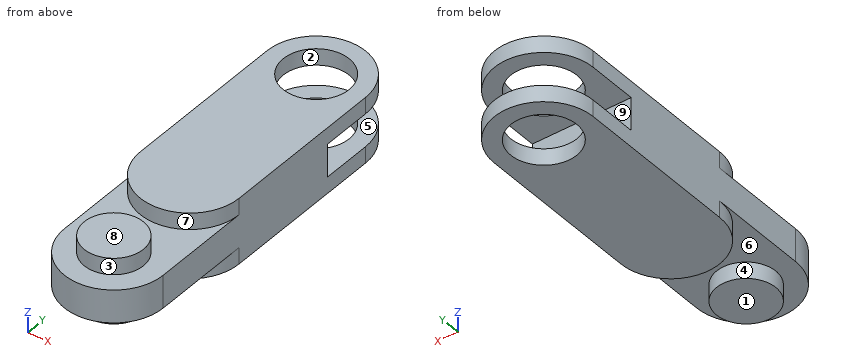
```python
from build123d import *

# Parameters (mm, degrees)
CROQUIS1_R                 = 10
SALIENTE_EXTRUIR1_DEPTH    = 10
CORTAR_EXTRUIR2_DEPTH      = 97.695398029
CORTAR_EXTRUIR2_DEPTH_BACK = 97.695398029
CROQUIS2_W                 = 10
CROQUIS2_H                 = 30
CORTAR_EXTRUIR4_START      = -5
CROQUIS4_R                 = 8.968507367
CORTAR_EXTRUIR4_DEPTH      = 92.695398029
CORTAR_EXTRUIR6_START      = 5
CROQUIS4_2_R               = 8.968507367
CORTAR_EXTRUIR6_DEPTH      = 92.695398029


with BuildPart() as part:
    # Croquis1 → Saliente-Extruir1 (new, symmetric)
    with BuildSketch(Plane.XY):
        with BuildLine():
            Line((-15, 0), (-15, 80))
            ThreePointArc((-15, 80), (0, 95), (15, 80))
            Line((15, 80), (15, 0))
            ThreePointArc((15, 0), (0, -15), (-15, 0))
        make_face()
        with Locations((0, 80)):
            Circle(CROQUIS1_R, mode=Mode.SUBTRACT)
    extrude(amount=SALIENTE_EXTRUIR1_DEPTH, both=True)

    # Croquis2 → Cortar-Extruir2 (cut, two sides: drawn at the far end of the back side and taken through both)
    with BuildSketch(Plane(origin=(0, 0, 0), x_dir=(0, 0, -1), z_dir=(1, 0, 0)).offset(-CORTAR_EXTRUIR2_DEPTH_BACK)):
        with Locations((0, 80)):
            Rectangle(CROQUIS2_W, CROQUIS2_H)
    extrude(amount=CORTAR_EXTRUIR2_DEPTH + CORTAR_EXTRUIR2_DEPTH_BACK, mode=Mode.SUBTRACT)

    # Croquis4 → Cortar-Extruir4 (cut, through all)
    with BuildSketch(Plane.XY.offset(CORTAR_EXTRUIR4_START)):
        with BuildLine():
            Line((-15, 30), (-15, 0))
            ThreePointArc((-15, 0), (0, -15), (15, 0))
            Line((15, 0), (15, 30))
            ThreePointArc((15, 30), (0, 15), (-15, 30))
        make_face()
        Circle(CROQUIS4_R, mode=Mode.SUBTRACT)
    extrude(amount=-CORTAR_EXTRUIR4_DEPTH, mode=Mode.SUBTRACT)

    # Croquis4<2> → Cortar-Extruir6 (cut, through all)
    with BuildSketch(Plane.XY.offset(CORTAR_EXTRUIR6_START)):
        with BuildLine():
            Line((-15, 30), (-15, 0))
            ThreePointArc((-15, 0), (0, -15), (15, 0))
            Line((15, 0), (15, 30))
            ThreePointArc((15, 30), (0, 15), (-15, 30))
        make_face()
        Circle(CROQUIS4_2_R, mode=Mode.SUBTRACT)
    extrude(amount=CORTAR_EXTRUIR6_DEPTH, mode=Mode.SUBTRACT)


solid = part.part
```
The listing builds one solid part. Answer for the finished solid, in the listing's coordinates (mm). Face numbers are marked on the shaded views. A direction names the side the tool comes from. Give positions to 0.01 mm unless a question says otherwise; leave off trailing zeros. Order: outer loops, then holes, each group sorted by start corner. A loop starts at its lowest first (then second) coordinate and runs counter-clockwise, first axis right, second up.
1) Find section B-B on x = 0. Write down the section's boundary in (y, z).
Reported:
outline: (-15, -5) - (-8.97, -5) - (-8.97, -10) - (8.97, -10) - (8.97, -5) - (15, -5) - (15, -10) - (70, -10) - (70, -5) - (65, -5) - (65, 5) - (70, 5) - (70, 10) - (15, 10) - (15, 5) - (8.97, 5) - (8.97, 10) - (-8.97, 10) - (-8.97, 5) - (-15, 5) - close; (90, -10) - (95, -10) - (95, -5) - (90, -5) - close; (90, 5) - (95, 5) - (95, 10) - (90, 10) - close
2) Determine the mould class of the marked faces 6, 7, 8 and 9 for opening direction Y: pulls with the +Y half, pulls with the -Y half, needs draft (parallel to the pull), parting line crosses it, or undercut.
Reported:
face 6: undercut
face 7: undercut
face 8: needs draft
face 9: pulls with the +Y half
3) Find section A-A on z = -6.25. Write down the section's boundary in (x, y).
Reported:
outline: (-15, 30) arc R15 ccw to (15, 30) - (15, 80) arc R15 ccw to (-15, 80) - close; circle Ø17.94 at (0, 0); hole circle Ø20 at (0, 80)
4) Given P1, Ø4, axis at x = -10, y = 3.5, coming from the +Z side; P2, Ø1, axis at x = 6.5, z = -2.5, coming from the +Y side; P3, Ø1, axis at x = 10, z = 6.5, coming from the +Y side; P4, Ø12, axis at x = 0, y = 80, coming from the -Z side, each flat-ended and moving along its own axis, determine where each tip first touches the part or whether it passes through.
Reported:
P1: stops at z = 10
P2: stops at y = 65
P3: stops at y = 91.61
P4: passes through
5) For the marked faces 1, 2, 3, 4 and 5, determine the directions among +Z, -Z, +X, -X, +Y, -Y from which every point of the face is accessible in a straight line to the end or side of a thin tool.
Reported:
face 1: -Z, +X, -X, +Y, -Y
face 2: +Z, -Z
face 3: +Z
face 4: -Z
face 5: +X, -X, +Y
6) Consider line 1 along Y through (x, z) = (0, 7); line 2 along X through (y, z) = (80, -6.8); line 3 along Z through (x, y) = (1.5, 90). Determine where each line is inside the solid, lowest interval first.
Reported:
line 1: y = -8.97 to 8.97, 15 to 70, 90 to 95
line 2: x = -15 to -10, 10 to 15
line 3: z = -10 to -5, 5 to 10
